```python
from build123d import *

# Parameters (mm, degrees)
ESQUISSE1_W             = 50
ESQUISSE1_H             = 57
ESQUISSE1_R             = 7
BOSS_EXTRU_1_DEPTH      = 8
ESQUISSE2_R             = 8
ENL_V_MAT_EXTRU_1_DEPTH = 5
ESQUISSE3_R             = 1.65
ENL_V_MAT_EXTRU_2_DEPTH = 10


with BuildPart() as part:
    # Esquisse1 → Boss.-Extru.1 (new body)
    with BuildSketch(Plane.XY):
        with Locations((25, 28.5)):
            Rectangle(ESQUISSE1_W, ESQUISSE1_H)
        with Locations((25, 20)):
            Circle(ESQUISSE1_R, mode=Mode.SUBTRACT)
    extrude(amount=BOSS_EXTRU_1_DEPTH)

    # Esquisse2 → Enlèv. mat.-Extru.1 (cut)
    with BuildSketch(Plane.XY.offset(8)):
        with Locations((25, 20)):
            Circle(ESQUISSE2_R)
    extrude(amount=-ENL_V_MAT_EXTRU_1_DEPTH, mode=Mode.SUBTRACT)

    # Esquisse3 → Enlèv. mat.-Extru.2 (cut)
    with BuildSketch(Plane(origin=(0, 57, 0), x_dir=(1, 0, 0), z_dir=(0, 1, 0))):
        with Locations((10, -4)):
            Circle(ESQUISSE3_R)
        with Locations((40, -4)):
            Circle(ESQUISSE3_R)
    extrude(amount=-ENL_V_MAT_EXTRU_2_DEPTH, mode=Mode.SUBTRACT)


solid = part.part
```
Can you work these out from the model? Positions are in its coordinate system, mm. A direction names the side the tool comes from. Round coordinates to 2 decimals unless told otherwise and drop trailing zeros. Loops run counter-clockwise (first coordinate to the right, second up) from the corner with the lowest first, then second, coordinate; pieces in that order, holes last. Notation, with made-up numbers: (57.5, 38) -> (82.5, 38) arc R33 cw to (82.5, 67) -> close; hole circle Ø6 at (55, 89.5). An arc over 180 degrees is marked (long way). Answer in a Markdown table with one row per item.
Item 1: Suppose I cut it at A-A, the plane y = 20. List the corners of the cut face in (x, z) for me, plus the area to 3 significant figures.
Answer block:
| item | result |
|---|---|
| outline | (0, 0) -> (18, 0) -> (18, 3) -> (17, 3) -> (17, 8) -> (0, 8) -> close; (32, 0) -> (50, 0) -> (50, 8) -> (33, 8) -> (33, 3) -> (32, 3) -> close |
| area | 278 mm² |
Item 2: Suppose I cut it at B-B, the plane x = 25. List the corners of the cut face in (y, z) for me.
Answer block:
| item | result |
|---|---|
| outline | (0, 0) -> (13, 0) -> (13, 3) -> (12, 3) -> (12, 8) -> (0, 8) -> close; (27, 0) -> (57, 0) -> (57, 8) -> (28, 8) -> (28, 3) -> (27, 3) -> close |
Item 3: Suppose I cut it at C-C, the plane z = 7.25. List the corners of the cut face in (x, y) for me.
Answer block:
| item | result |
|---|---|
| outline | (0, 0) -> (50, 0) -> (50, 57) -> (0, 57) -> close; hole circle Ø16 at (25, 20) |
Item 4: Suppose I cut it at D-D, the plane y = 52. List the corners of the cut face in (x, z) for me.
Answer block:
| item | result |
|---|---|
| outline | (0, 0) -> (50, 0) -> (50, 8) -> (0, 8) -> close; hole circle Ø3.3 at (10, 4); hole circle Ø3.3 at (40, 4) |
Item 5: On a 3-axis mill with a long thin cutter (end or side, diameter ignored), from which of +Z, -Z, +X, -X, +Y, -Y can I reach the whole of each face in a straight line? I mean faces 1 (the cylindrical face through (17, 20, 6)), 2 (the flat face through (25, 29, 8)), 3 (the flat face through (40, 47, 4)). Say none if no direction works.
Answer block:
| item | result |
|---|---|
| face 1 | +Z |
| face 2 | +Z, +X, -X, +Y, -Y |
| face 3 | +Y |
Item 6: Will these pins go through, and if not, where does the flat tip stop? P1, Ø2.5, axis at x = 40, z = 3.5, coming from the +Y side; P2, Ø3, axis at x = 40, z = 4, coming from the +Y side.
Answer block:
| item | result |
|---|---|
| P1 | y = 57 |
| P2 | y = 47 |
Item 7: We'd pull the mould along Z, two halves only. Please class faces 4 (the cylindrical face through (23.483, 13.166, 1.479)), 5 (the cylindrical face through (38.35, 52.07, 3.93)), 6 (the flat face through (25, 29, 0)): released by +Z, released by -Z, zero draft, split by the parting line, or undercut.
Answer block:
| item | result |
|---|---|
| face 4 | zero draft |
| face 5 | undercut |
| face 6 | released by -Z |
Item 8: If I drill on probe 1 along X at (y, z) = (52.75, 4); probe 2 along Y at (x, z) = (25, 5.15); probe 3 along Y at (x, z) = (25, 0.7), over which ranges is the centre line in solid material (lowest first)?
Answer block:
| item | result |
|---|---|
| probe 1 | 0 to 8.35, 11.65 to 38.35, 41.65 to 50 |
| probe 2 | 0 to 12, 28 to 57 |
| probe 3 | 0 to 13, 27 to 57 |
